```python
from build123d import *

# Parameters (mm, degrees)
PAD_DEPTH       = 2
SKETCH001_W     = 35
SKETCH001_H     = 2
PAD001_DEPTH    = 18
SKETCH002_W     = 44
SKETCH002_H     = 2
PAD002_DEPTH    = 24
CHAMFER_1_SIZE2 = 17.99
CHAMFER_1_SIZE  = 4.49
CHAMFER_2_SIZE2 = 17.99
CHAMFER_2_SIZE  = 4.49
FILLET_R        = 3
SKETCH003_R     = 1.25
POCKET_DEPTH    = 5


with BuildPart() as part:
    # Sketch → Pad (new body)
    with BuildSketch(Plane.XY):
        Polygon((-17.5, -15), (17.5, -15), (17.5, -7), (11, 7), (-11, 7), (-17.5, -7), align=None)
    extrude(amount=PAD_DEPTH)

    # Sketch001 (on Face8 of Pad) → Pad001 (join)
    with BuildSketch(Plane.XY.offset(2)):
        with Locations((0, -14)):
            Rectangle(SKETCH001_W, SKETCH001_H)
    extrude(amount=PAD001_DEPTH)

    # Sketch002 (on Face12 of Pad001) → Pad002 (join)
    with BuildSketch(Plane.XY.offset(20)):
        with Locations((0, -14)):
            Rectangle(SKETCH002_W, SKETCH002_H)
    extrude(amount=PAD002_DEPTH)

    # Chamfer 1
    chamfer_1_edges = [part.edges().sort_by_distance(p)[0] for p in [
        (-17.5, -14, 20),
    ]]
    chamfer_1_side = part.faces().sort_by_distance((-19.75, -14, 20))[0]
    chamfer(chamfer_1_edges, length=CHAMFER_1_SIZE, length2=CHAMFER_1_SIZE2, reference=chamfer_1_side)

    # Chamfer 2
    chamfer_2_edges = [part.edges().sort_by_distance(p)[0] for p in [
        (17.5, -14, 20),
    ]]
    chamfer_2_side = part.faces().sort_by_distance((19.75, -14, 20))[0]
    chamfer(chamfer_2_edges, length=CHAMFER_2_SIZE, length2=CHAMFER_2_SIZE2, reference=chamfer_2_side)

    # Fillet
    fillet_edges = [part.edges().sort_by_distance(p)[0] for p in [
        (22, -14, 44),
        (17.5, -7, 1),
        (11, 7, 1),
        (-11, 7, 1),
        (-17.5, -7, 1),
        (-22, -14, 44),
    ]]
    fillet(fillet_edges, radius=FILLET_R)

    # Sketch003 (on Face1 of Fillet) → Pocket (cut)
    with BuildSketch(Plane(origin=(0, -13, 0), x_dir=(-1, 0, 0), z_dir=(0, 1, 0))):
        with Locations((-19.5, 39)):
            Circle(SKETCH003_R)
        with Locations((19.5, 23)):
            Circle(SKETCH003_R)
    extrude(amount=-POCKET_DEPTH, mode=Mode.SUBTRACT)


solid = part.part
```
CAD build for the part. Positions are in the model's coordinates, mm. A direction names the side the tool comes from. Coordinates: 2 decimals unless noted, no trailing zeros. Loops run counter-clockwise (first coordinate to the right, second up) from the corner with the lowest first, then second, coordinate; pieces in that order, holes last. Notation, with made-up numbers: (-3.75, 32.25) - (33.25, 32.25) arc R29 cw to (33.25, 65.25) - close; hole circle Ø1 at (-13.75, -26.75). An arc over 180 degrees is marked (long way). Use CSV: the item, a comma, the result in double quotes. Start each with the question number.
Q1. Cut at A-A, the plane z = 23. List the corners of the cut face in (x, y), then the cut area to 3 significant figures.
Q2. Cut at C-C, the plane y = -9.25. List the corners of the cut face in (x, z), then the cut area to 3 significant figures.
Q3. Cut at B-B, the plane x = 1. List the corners of the cut face in (y, z).
Q4. Probe probe 1 along Y at (x, z) = (16, 33); probe 2 along Z at (x, y) = (14.5, -1). List the from-to ranges inside material, lowest first. Write a range as from..to.
Q5. Drop flat-ended pins along their axis: P1, Ø10, axis at x = 5.5, y = -2.5, coming from the +Z side; P2, Ø12.5, axis at x = -2.5, z = 25, coming from the +Y side; P3, Ø1, axis at y = -13, z = 1.5, coming from the -X side. Give the stop position or say it passes through.
Q6. Cut at D-D, the plane z = 6.5. List the corners of the cut face in (x, y), then the cut area to 3 significant figures.
Q7. Two-plate mould, pull along X, no slides. Class faces 3 (the cylindrical face through (-20.655, -13.986, 22.521)), 4 (the cylindrical face through (-10.68, 6.54, 1.01)), 5 (the flat face through (0, -13, 23)), 6 (the flat face through (17.5, -11, 1)): +X half, -X half, draft (parallel to the pull), parting line (faces both ways), or undercut.
Q8. 3-axis set-ups, long thin cutter, end or side, ignore diameter. For faces 1 (the flat face through (-14.476, -0.486, 0.986)), 2 (the flat face through (0, -3, 2)): which of +Z, -Z, +X, -X, +Y, -Y reach the whole face in a straight line?
Here are the results:
1,outline,"(-22, -15) - (-20.75, -15) - (-20.75, -13) - (-22, -13) - close; (-18.25, -15) - (22, -15) - (22, -13) - (-18.25, -13) - close"
1,area,"83.0 mm2"
2,outline,"(-17.5, 0) - (17.5, 0) - (17.5, 2) - (-17.5, 2) - close"
2,area,"70.0 mm2"
3,outline,"(-15, 0) - (7, 0) - (7, 2) - (-13, 2) - (-13, 44) - (-15, 44) - close"
4,probe 1,"-15..-13"
4,probe 2,"0..2"
5,P1,"z = 2"
5,P2,"y = -13"
5,P3,"x = -17.5"
6,outline,"(-18.62, -15) - (18.62, -15) - (18.62, -13) - (-18.62, -13) - close"
6,area,"74.5 mm2"
7,face 3,"undercut"
7,face 4,"-X half"
7,face 5,"draft"
7,face 6,"+X half"
8,face 1,"+Z, -Z, -X, +Y"
8,face 2,"+Z, +X, -X, +Y"
